from build123d import *

# Parameters (mm, degrees)
SKETCH1_W           = 57
SKETCH1_H           = 57
BOSS_EXTRUDE2_DEPTH = 56
CUT_EXTRUDE1_DEPTH  = 50
FILLET1_R           = 2.54
SKETCH3_R           = 2.499995
CUT_EXTRUDE2_DEPTH  = 25.4
SKETCH4_R           = 19.05
BOSS_EXTRUDE3_DEPTH = 1.6
FILLET2_R           = 0.5
SKETCH5_R           = 3.175
BOSS_EXTRUDE4_DEPTH = 21
CUT_EXTRUDE4_DEPTH  = 15


with BuildPart() as part:
    # Sketch1 → Boss-Extrude2 (new body)
    with BuildSketch(Plane(origin=(0, 0, 0), x_dir=(1, 0, 0), z_dir=(0, 1, 0))):
        Rectangle(SKETCH1_W, SKETCH1_H)
    extrude(amount=BOSS_EXTRUDE2_DEPTH)

    # Sketch2 → Cut-Extrude1 (cut)
    with BuildSketch(Plane.XZ):
        with BuildLine():
            Line((28.5, -18.5), (28.5, -28.5))
            Line((28.5, -28.5), (18.5, -28.5))
            ThreePointArc((18.5, -28.5), (21.428932188, -21.428932188), (28.5, -18.5))
        make_face()
        with BuildLine():
            Line((-28.5, -28.5), (-28.5, -18.5))
            ThreePointArc((-28.5, -18.5), (-21.428932188, -21.428932188), (-18.5, -28.5))
            Line((-18.5, -28.5), (-28.5, -28.5))
        make_face()
        with BuildLine():
            Line((-28.5, 28.5), (-18.5, 28.5))
            ThreePointArc((-18.5, 28.5), (-21.428932188, 21.428932188), (-28.5, 18.5))
            Line((-28.5, 18.5), (-28.5, 28.5))
        make_face()
        with BuildLine():
            Line((28.5, 28.5), (28.5, 18.5))
            ThreePointArc((28.5, 18.5), (21.428932188, 21.428932188), (18.5, 28.5))
            Line((18.5, 28.5), (28.5, 28.5))
        make_face()
    extrude(amount=-CUT_EXTRUDE1_DEPTH, mode=Mode.SUBTRACT)

    # Fillet1
    fillet1_edges = [part.edges().sort_by_distance(p)[0] for p in [
        (-28.5, 53, -28.5),
        (28.5, 53, -28.5),
        (28.5, 53, 28.5),
        (-28.5, 53, 28.5),
    ]]
    fillet(fillet1_edges, radius=FILLET1_R)

    # Sketch3 → Cut-Extrude2 (cut)
    with BuildSketch(Plane(origin=(0, 56, 0), x_dir=(1, 0, 0), z_dir=(0, 1, 0))):
        with Locations((-23.50001, -23.50001)):
            Circle(SKETCH3_R)
        with Locations((-23.50001, 23.50001)):
            Circle(SKETCH3_R)
        with Locations((23.50001, 23.50001)):
            Circle(SKETCH3_R)
        with Locations((23.50001, -23.50001)):
            Circle(SKETCH3_R)
    extrude(amount=-CUT_EXTRUDE2_DEPTH, mode=Mode.SUBTRACT)

    # Sketch4 → Boss-Extrude3 (add)
    with BuildSketch(Plane(origin=(0, 56, 0), x_dir=(1, 0, 0), z_dir=(0, 1, 0))):
        Circle(SKETCH4_R)
    extrude(amount=BOSS_EXTRUDE3_DEPTH)

    # Fillet2
    fillet2_edges = [part.edges().sort_by_distance(p)[0] for p in [
        (-19.05, 56, 0),
    ]]
    fillet(fillet2_edges, radius=FILLET2_R)

    # Sketch5 → Boss-Extrude4 (add)
    with BuildSketch(Plane(origin=(0, 57.6, 0), x_dir=(1, 0, 0), z_dir=(0, 1, 0))):
        Circle(SKETCH5_R)
    extrude(amount=BOSS_EXTRUDE4_DEPTH)

    # Sketch6 → Cut-Extrude4 (cut)
    with BuildSketch(Plane(origin=(0, 78.6, 0), x_dir=(1, 0, 0), z_dir=(0, 1, 0))):
        with BuildLine():
            Line((1.710263138, -2.675), (-1.710263138, -2.675))
            ThreePointArc((-1.710263138, -2.675), (0, -3.175), (1.710263138, -2.675))
        make_face()
    extrude(amount=-CUT_EXTRUDE4_DEPTH, mode=Mode.SUBTRACT)


solid = part.part
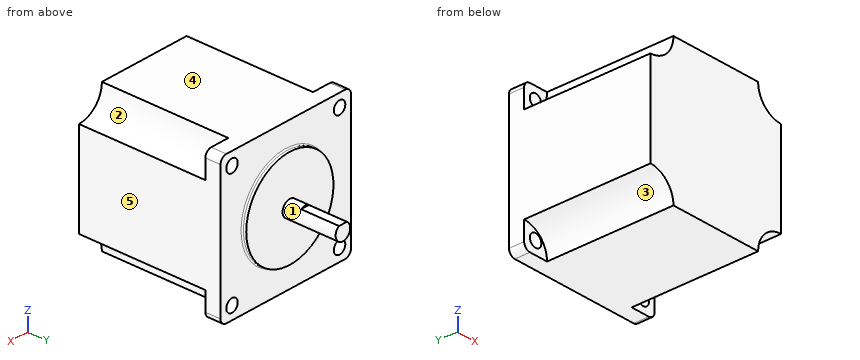
Source: CAD feature listing. Evaluate the final solid. Frame: model axes, mm. Face numbers are marked on the shaded views. A direction names the side the tool comes from. Give positions to 0.01 mm unless a question says otherwise; leave off trailing zeros. Write each loop counter-clockwise with the first axis right and the second up, starting at its lowest first coordinate (ties: lowest second). Pieces come first, ordered by that corner, then holes. Notation, with made-up numbers: (78.5, 43) -> (124.5, 43) arc R27 ccw to (124.5, 60) -> close; hole circle Ø5 at (38.25, 25). An arc over 180 degrees is marked (long way). Return JSON: item names as keys, results as strings. Group by question number.
1. Section B-B, the plane y = 51.5. Output: boundary loops of the cut face in (x, z).
2. Access query for the marked faces 1, 2, 3, 4 and 5. Directions: +Z, -Z, +X, -X, +Y, -Y. A direction counts if a zero-diameter tool reaches every point of the face in a straight line with its end or side. Return the directions, or none.
3. Material intervals for line 1 (X direction, y = 53, z = 25.5); line 2 (Y direction, x = 4, z = -10); line 3 (Y direction, x = -21.5, z = -9), sorted ascending. Write a range as from..to.
4. Section C-C, the plane z = 0. Output: boundary loops of the cut face in (x, y) (3 decimals), then the cut area to 3 significant figures.
5. Pin query (flat end, axial travel): pin 1 Ø3 at (x, z) = (23.5, -23.5) entering from +Y; pin 2 Ø5 at (x, z) = (-22.5, -25.5) entering from -Y; pin 3 Ø6.5 at (x, z) = (-23.5, -23.5) entering from +Y; pin 4 Ø4 at (x, y) = (-0.5, 74) entering from +Z (3 decimals). Return the tip coordinate at first contact, or that it passes through.
6. Section D-D, the plane y = 39. Output: boundary loops of the cut face in (x, z).
7. Section A-A, the plane x = -22.5. Output: boundary loops of the cut face in (y, z), then the cut area to 3 significant figures.
Determined:
{
 "1": {"outline": "(-28.5, -25.96) arc R2.54 ccw to (-25.96, -28.5) -> (25.96, -28.5) arc R2.54 ccw to (28.5, -25.96) -> (28.5, 25.96) arc R2.54 ccw to (25.96, 28.5) -> (-25.96, 28.5) arc R2.54 ccw to (-28.5, 25.96) -> close; hole circle Ø5 at (-23.5, -23.5); hole circle Ø5 at (-23.5, 23.5); hole circle Ø5 at (23.5, -23.5); hole circle Ø5 at (23.5, 23.5)"},
 "2": {"face 1": "+Y", "face 2": "+Z, +X, -Y", "face 3": "-Z, -X, -Y", "face 4": "+Z, +X, -X, +Y, -Y", "face 5": "+Z, -Z, +X, +Y, -Y"},
 "3": {"line 1": "x = -28.5..-25, -22..22, 25..28.5", "line 2": "y = 0..57.6", "line 3": "y = 0..56"},
 "4": {"outline": "(-28.5, 0) -> (28.5, 0) -> (28.5, 56) -> (19.55, 56) arc R0.5 cw to (19.05, 56.5) -> (19.05, 57.6) -> (3.175, 57.6) -> (3.175, 78.6) -> (-3.175, 78.6) -> (-3.175, 57.6) -> (-19.05, 57.6) -> (-19.05, 56.5) arc R0.5 cw to (-19.55, 56) -> (-28.5, 56) -> close", "area": "3,390 mm2"},
 "5": {"pin 1": "passes through", "pin 2": "stops at y = 50", "pin 3": "stops at y = 56", "pin 4": "stops at z = 2.675"},
 "6": {"outline": "(-28.5, -18.5) arc R10 cw to (-18.5, -28.5) -> (18.5, -28.5) arc R10 cw to (28.5, -18.5) -> (28.5, 18.5) arc R10 cw to (18.5, 28.5) -> (-18.5, 28.5) arc R10 cw to (-28.5, 18.5) -> close"},
 "7": {"outline": "(0, -20.5) -> (50, -20.5) -> (50, -21.21) -> (56, -21.21) -> (56, 21.21) -> (50, 21.21) -> (50, 20.5) -> (0, 20.5) -> close; (50, -28.5) -> (56, -28.5) -> (56, -25.79) -> (50, -25.79) -> close; (50, 25.79) -> (56, 25.79) -> (56, 28.5) -> (50, 28.5) -> close", "area": "2,340 mm2"}
}
